Geometry check sheet. Reference: the model listing, model coordinates, mm. Give positions to 0.01 mm unless a question says otherwise; leave off trailing zeros. Write each loop counter-clockwise with the first axis right and the second up, starting at its lowest first coordinate (ties: lowest second). Pieces come first, ordered by that corner, then holes. Notation, with made-up numbers: (64, 57.25) -> (97, 57.25) arc R19 cw to (97, 65.25) -> close; hole circle Ø6 at (57.5, -18.5). An arc over 180 degrees is marked (long way). Use a Markdown table: item, result. Add a question column.
from build123d import *

# Parameters (mm, degrees)
SKETCH1_W        = 38.1
SKETCH1_H        = 482.6
EXTRUSION1_DEPTH = 3.175
HOLE1_D          = 6.35
HOLE2_D          = 12.7
EXTRUSION2_START = -3.175
SKETCH6_R        = 6.35
EXTRUSION2_DEPTH = 3.175
HOLE3_D          = 12.7
HOLE4_D          = 3.96875
EXTRUSION3_START = -3.175
SKETCH11_R       = 1.984375
EXTRUSION3_DEPTH = 3.175


with BuildPart() as part:
    # Sketch1 → Extrusion1 (new body)
    with BuildSketch(Plane(origin=(0, 0, 0), x_dir=(-1, 0, 0), z_dir=(0, 1, 0))):
        Rectangle(SKETCH1_W, SKETCH1_H)
    extrude(amount=EXTRUSION1_DEPTH)

    # Hole1 (through all)
    with Locations(Plane(origin=(0, 3.175, 0), x_dir=(1, 0, 0), z_dir=(0, 1, 0))):
        with Locations((0, -228.6), (0, 228.6), (0, 0)):
            Hole(HOLE1_D / 2)

    # Hole2 (through all)
    with Locations(Plane(origin=(0, 3.175, 0), x_dir=(1, 0, 0), z_dir=(0, 1, 0))):
        with Locations((0, -101.6), (0, 101.6)):
            Hole(HOLE2_D / 2)

    # Sketch6 → Extrusion2 (add)
    with BuildSketch(Plane(origin=(0, 3.175, 0), x_dir=(1, 0, 0), z_dir=(0, 1, 0)).offset(EXTRUSION2_START)):
        with Locations((0, -101.6)):
            Circle(SKETCH6_R)
        with Locations((0, 101.6)):
            Circle(SKETCH6_R)
    extrude(amount=EXTRUSION2_DEPTH)

    # Hole3 (through all)
    with Locations(Plane(origin=(0, 3.175, 0), x_dir=(1, 0, 0), z_dir=(0, 1, 0))):
        with Locations((0, 114.3), (0, -114.3)):
            Hole(HOLE3_D / 2)

    # Hole4 (through all)
    with Locations(Plane(origin=(0, 3.175, 0), x_dir=(1, 0, 0), z_dir=(0, 1, 0))):
        with Locations((0, -88.9), (0, -139.7), (0, 88.9), (0, 139.7)):
            Hole(HOLE4_D / 2)

    # Sketch11 → Extrusion3 (add)
    with BuildSketch(Plane(origin=(0, 3.175, 0), x_dir=(1, 0, 0), z_dir=(0, 1, 0)).offset(EXTRUSION3_START)):
        with Locations((0, 88.9)):
            Circle(SKETCH11_R)
        with Locations((0, -88.9)):
            Circle(SKETCH11_R)
        with Locations((0, -139.7)):
            Circle(SKETCH11_R)
        with Locations((0, 139.7)):
            Circle(SKETCH11_R)
    extrude(amount=EXTRUSION3_DEPTH)


solid = part.part
1) Sectioned sample at B-B, the plane z = -114.3. Enter the section's corners in (x, y) (3 decimals).
2) Material ranges on probe 1 along Z at (x, y) = (0, 1.65) (3 decimals); probe 2 along Z at (x, y) = (-0.5, 2); probe 3 along X at (y, z) = (2.25, 228.6) (3 decimals), recorded low to high. Write a range as [from, to].
3) Draft check along X on faces 1 (the face through (0.3, 3.175, 3.4)), 2 (the face through (-3.414, 1.565, 108.946)), 3 (the face through (1.38, 1.57, -108.1)). Enter one of: +X half, -X half, draft (parallel to the pull), parting line (faces both ways), or undercut.
4) Gauge pin test, flat end, axial feed: P1, Ø4, axis at x = 0, z = -228.6, coming from the -Y side. Record the tip position at first contact, or that the pin passes through.
5) Sectioned sample at A-A, the plane y = 0.75. Enter the section's corners in (x, z) (3 decimals).
Check values:
| question | item | result |
|---|---|---|
| 1 | outline | (-19.05, 0) -> (-6.35, 0) -> (-6.35, 3.175) -> (-19.05, 3.175) -> close; (6.35, 0) -> (19.05, 0) -> (19.05, 3.175) -> (6.35, 3.175) -> close |
| 2 | probe 1 | [-241.3, -231.775], [-225.425, -120.65], [-107.95, -3.175], [3.175, 107.95], [120.65, 225.425], [231.775, 241.3] |
| 2 | probe 2 | [-241.3, -231.74], [-225.46, -120.63], [-107.97, -3.14], [3.14, 107.97], [120.63, 225.46], [231.74, 241.3] |
| 2 | probe 3 | [-19.05, -3.175], [3.175, 19.05] |
| 3 | face 1 | draft |
| 3 | face 2 | undercut |
| 3 | face 3 | undercut |
| 4 | P1 | through |
| 5 | outline | (-19.05, -241.3) -> (19.05, -241.3) -> (19.05, 241.3) -> (-19.05, 241.3) -> close; hole circle Ø12.7 at (0, -114.3); hole circle Ø12.7 at (0, 114.3); hole circle Ø6.35 at (0, -228.6); hole circle Ø6.35 at (0, 0); hole circle Ø6.35 at (0, 228.6) |
